Check sheet for the drawn part. Datum: minimum x, y, z corner. Units: mm. A direction names the side the tool comes from. Coordinates: 2 decimals unless noted, no trailing zeros. Loops run counter-clockwise (first coordinate to the right, second up) from the corner with the lowest first, then second, coordinate; pieces in that order, holes last.
Q1. Go/stop test with flat-tipped pins: P1, Ø2, axis at y = 6, z = 2.5, coming from the -X side; P2, Ø6, axis at y = 5, z = 4.5, coming from the +X side; P3, Ø5, axis at x = 5.5, z = 4, coming from the +Y side; P4, Ø3, axis at x = 6, y = 6, coming from the -Z side. Record where each tip stops, or that it passes through.
Q2. Access from +Z, -Z, +X, -X, +Y, -Y to the whole of each face (thin tool, end or side, straight path). Record for the marked faces 1 and 2.
Q3. Mould release check, pull along Z, two halves, no side actions. Record for the marked faces 3, 4 and 5: +Z half, -Z half, draft (parallel to the pull), parting line (faces both ways), or undercut.
Q4. Sectioned sample at A-A (y = 7.25). Enter the section's corners in (x, z), then the cut area to 3 significant figures.
Q5. Sectioned sample at C-C (y = 1.5). Enter the section's corners in (x, z), then the cut area to 3 significant figures.
Q6. Sectioned sample at B-B (x = 9.75). Enter the section's corners in (y, z).
Q7. Material ranges on probe 1 along X at (y, z) = (6.5, 5); probe 2 along Y at (x, z) = (8.75, 8.5); probe 3 along Z at (x, y) = (7.5, 7), recorded low to high.
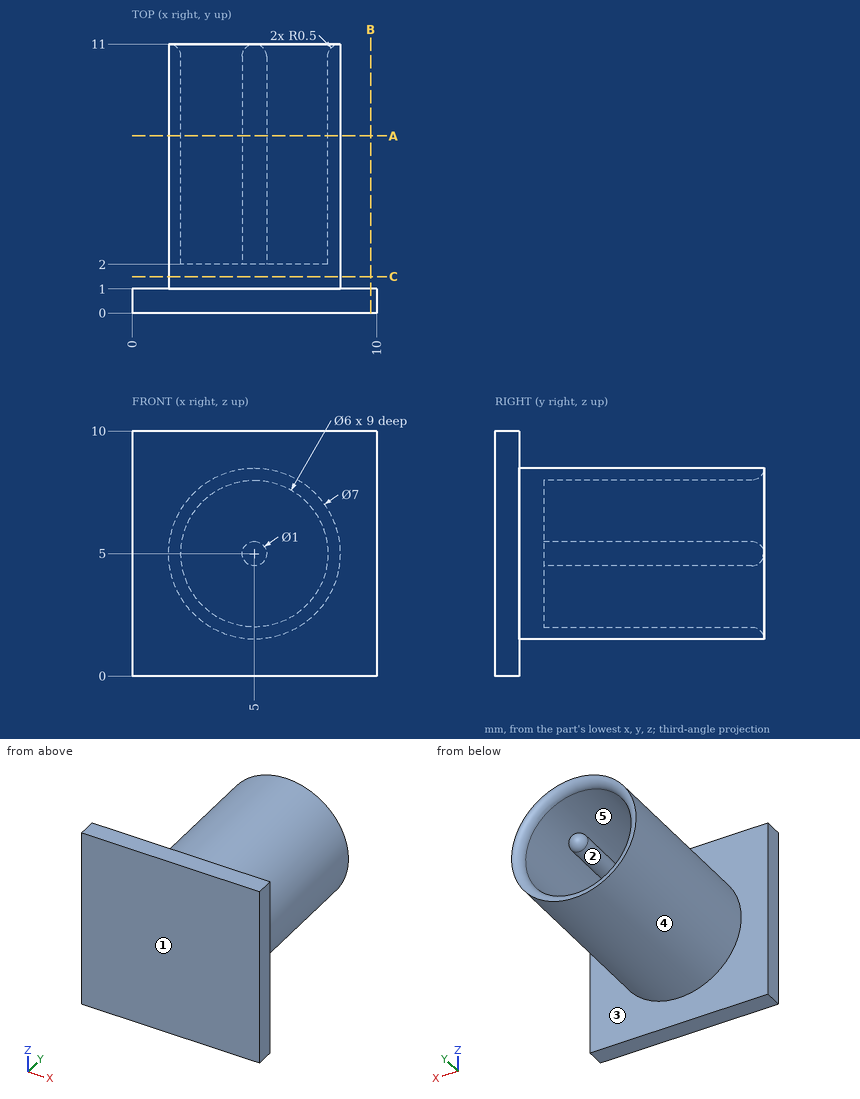
Geometry check:
1. P1: stops at x = 1.84
1. P2: stops at x = 8.5
1. P3: stops at y = 11
1. P4: stops at z = 1.5
2. face 1: +Z, -Z, +X, -X, -Y
2. face 2: +Y
3. face 3: draft
3. face 4: parting line
3. face 5: undercut
4. outline: circle Ø7 at (5, 5); circle Ø1 at (5, 5); hole circle Ø6 at (5, 5)
4. area: 11.0 mm2
5. outline: circle Ø7 at (5, 5)
5. area: 38.5 mm2
6. outline: (0, 0) - (1, 0) - (1, 10) - (0, 10) - close
7. probe 1: x = 1.5 to 2, 4.5 to 5.5, 8 to 8.5
7. probe 2: y = 0 to 1
7. probe 3: z = 2.55 to 3.34, 6.66 to 7.45
